Geometry check sheet. Reference: drawing and pictorial views, mm from the part's lowest x, y, z. Give positions to 0.01 mm unless a question says otherwise; leave off trailing zeros. Loops run counter-clockwise (first coordinate to the right, second up) from the corner with the lowest first, then second, coordinate; pieces in that order, holes last. Notation, with made-up numbers: M 7,27.5 L 24,27.5 A20 cw 24,46.5 Z; hole C -3.5,-6 d9. An arc over 180 degrees is marked long. Put each result on its own line as item: value. Start each with the question number.
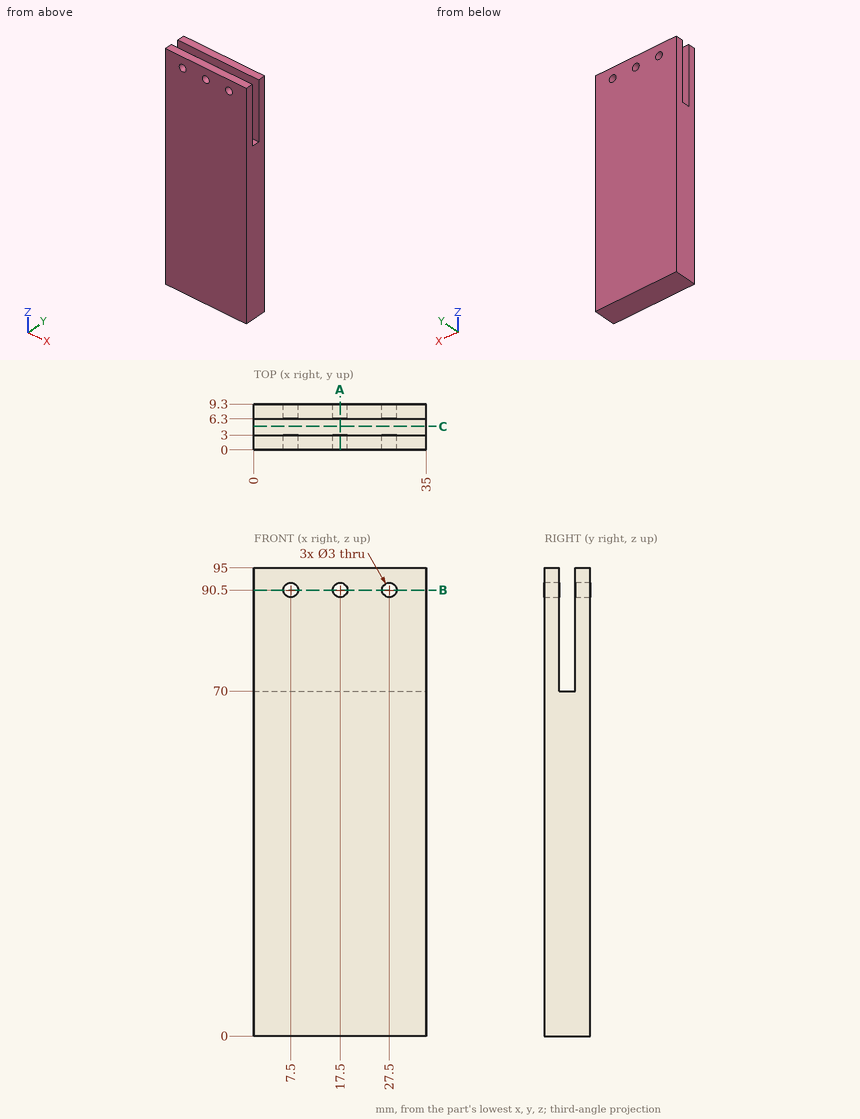
Q1. Depth check by flat-ended pin: P1, Ø1.5, axis at x = 18.5, z = 22, coming from the -Y side. Enter the tip coordinate at first touch or a pass-through.
Q2. Thickness scan on line 1 along X through (y, z) = (7.6, 90.5); line 2 along Y through (x, z) = (24, 82); line 3 along Z through (x, y) = (17, 1.5). Record the ranges inside material, lowest first. Write a range as [from, to].
Q3. Section check A-A, the plane x = 17.5. Record the cut outline in (y, z), then the cut area to 3 significant figures.
Q4. Section check C-C, the plane y = 4.75. Record the cut outline in (x, z).
Q5. Section check B-B, the plane z = 90.5. Give the number of separate pieces and of enclosed holes in the cut face, then the cut area to 3 significant figures.
Found:
1. P1: stops at y = 0
2. line 1: x = [0, 6], [9, 16], [19, 26], [29, 35]
2. line 2: y = [0, 3], [6.3, 9.3]
2. line 3: z = [0, 89.09], [91.91, 95]
3. outline: M 0,0 L 9.3,0 L 9.3,89 L 6.3,89 L 6.3,70 L 3,70 L 3,89 L 0,89 Z; M 0,92 L 3,92 L 3,95 L 0,95 Z; M 6.3,92 L 9.3,92 L 9.3,95 L 6.3,95 Z
3. area: 783 mm^2
4. outline: M 0,0 L 35,0 L 35,70 L 0,70 Z
5. separate pieces: 8
5. enclosed holes: 0
5. area: 156 mm^2
